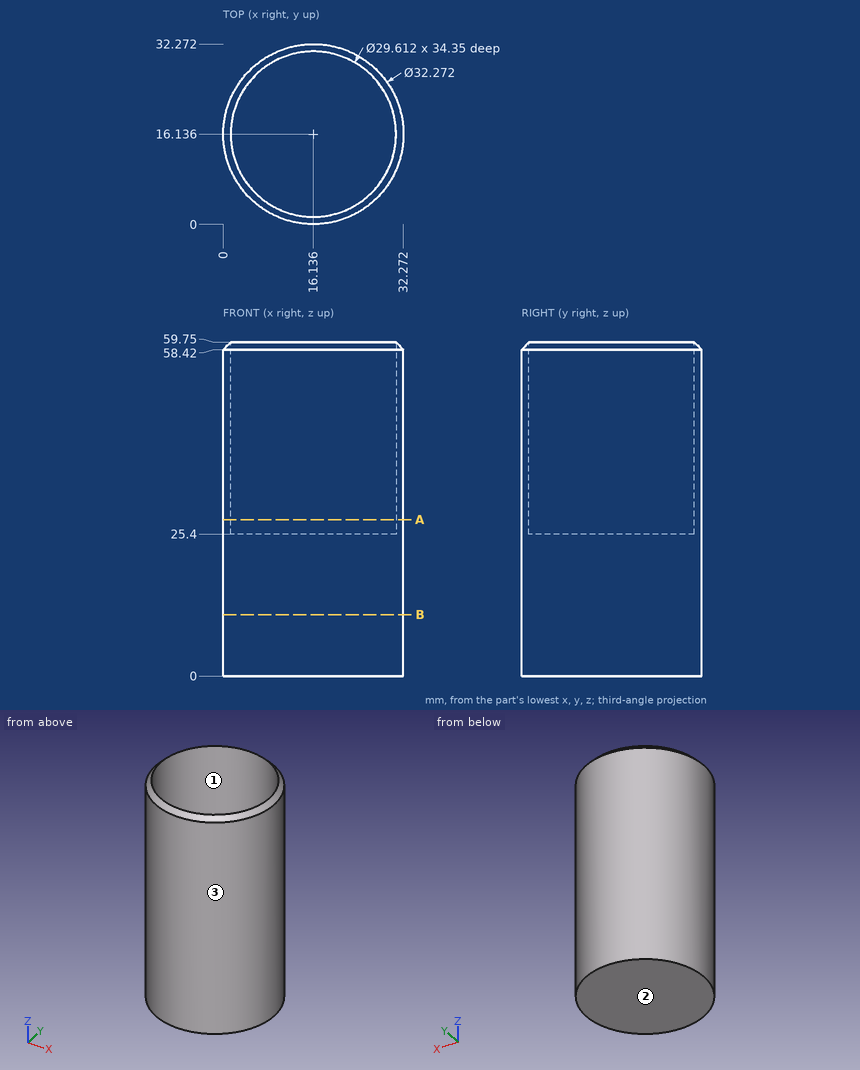
Verification items for this drawing (mm, ordinates from the low corner). Coordinates: 2 decimals unless noted, no trailing zeros. Write each loop counter-clockwise with the first axis right and the second up, starting at its lowest first coordinate (ties: lowest second). Pieces come first, ordered by that corner, then holes. Notation, with made-up numbers: (52.25, -22.75) -> (88.25, -22.75) arc R14 cw to (88.25, -9.75) -> close; hole circle Ø3 at (35, 43.25). An arc over 180 degrees is marked (long way). One line per item, written item: value. Start each with the question number.
Q1. Cross-section at B-B on z = 11. Enter the section's corners in (x, y).
Q2. Thickness scan on L1, parallel to Z at x = 5, y = 24; L2, parallel to Y at x = 24, z = 46 (1 decimal); L3, parallel to Y at x = 15, z = 55.5. Record the ranges inside material, lowest first. Write a range as from..to.
Q3. Go/stop test with flat-tipped pins: P1, Ø12, axis at x = 8, z = 10, coming from the +Y side; P2, Ø3, axis at x = 14, y = 26.5, coming from the +Z side; P3, Ø2, axis at x = 17, z = 11.5, coming from the -Y side; P4, Ø8, axis at x = 5.5, z = 39, coming from the +Y side (1 decimal). Record where each tip stops, or that it passes through.
Q4. Cross-section at A-A on z = 28. Enter the section's corners in (x, y).
Q5. Mould release check, pull along X, two halves, no side actions. Record for the marked faces 1, 2 and 3: pulls with the +X half, pulls with the -X half, needs draft (parallel to the pull), parting line crosses it, or undercut.
Checked values:
1. outline: circle Ø32.27 at (16.14, 16.14)
2. L1: z = 0..25.4
2. L2: y = 2..3.6, 28.7..30.2
2. L3: y = 0.04..1.37, 30.9..32.23
3. P1: stops at y = 32.13
3. P2: stops at z = 25.4
3. P3: stops at y = 0
3. P4: stops at y = 30.8
4. outline: circle Ø32.27 at (16.14, 16.14); hole circle Ø29.61 at (16.14, 16.14)
5. face 1: undercut
5. face 2: needs draft
5. face 3: parting line crosses it
